Part model, mm, in its own coordinate system. A direction names the side the tool comes from. Round coordinates to 2 decimals unless told otherwise and drop trailing zeros. Write each loop counter-clockwise with the first axis right and the second up, starting at its lowest first coordinate (ties: lowest second). Pieces come first, ordered by that corner, then holes. Notation, with made-up numbers: M 32,81 L 41,81 A11 ccw 41,90 Z; hole C 26,-16.5 d10. An arc over 180 degrees is marked long. One line per question, with ' | ' between items. Start each with the question number.
1) Tool access for faces 4 (the face through (6.46, 2.75, 0.99)), 5 (the face through (0, 2, 1)), 6 (the face through (7.5, 5, 1)): list every direction of +Z, -Z, +X, -X, +Y, -Y with a clear straight run to the whole face (end or side of a thin tool).
2) Saw through at B-B (y = 4). List the corners of the cut face in (x, z).
3) Drop flat-ended pins along their axis: pin 1 Ø0.5 at (y, z) = (5.5, 0.5) entering from +X; pin 2 Ø0.6 at (x, z) = (-0.5, 1) entering from -Y; pin 3 Ø1.1 at (y, z) = (5.5, 1.5) entering from -X; pin 4 Ø1.5 at (x, y) = (-6.5, 4) entering from +Z. Give the stop position or say it passes through.
4) Wall check: probe 1 along X at (y, z) = (4, 1.45); probe 2 along X at (y, z) = (3.2, 1.5); probe 3 along Y at (x, z) = (-2.75, 1.85). Give the ranges that are in metal, low to high. Write a range as [from, to].
5) Saw through at D-D (x = 3.5). List the corners of the cut face in (y, z).
6) Mould opens along X. For faces 1 (the face through (-3.75, 1, 1)), 2 (the face through (0, 3, 2)), 3 (the face through (9.699, 5.465, 1.014)) say: pulls with the +X half, pulls with the -X half, needs draft (parallel to the pull), parting line crosses it, or undercut.
7) Saw through at A-A (y = 1.35). List the corners of the cut face in (x, z).
8) Saw through at C-C (z = 1.15). List the corners of the cut face in (x, y).
```python
from build123d import *

# Parameters (mm, degrees)
TUBE_PLATE_BODY_DEPTH   = 2
TUBE_PLATE_CONTOURING_R = 1


with BuildPart() as part:
    # Sketch1 → Tube Plate Body (new body)
    with BuildSketch(Plane.XY):
        with BuildLine():
            Line((-10, 0), (-10, 5.75))
            Line((-10, 5.75), (-7.5, 5.75))
            Line((-7.5, 5.75), (-7.5, 4.75))
            ThreePointArc((-7.5, 4.75), (-6.5, 2.75), (-5.5, 4.75))
            Line((-5.5, 4.75), (-5.5, 5.75))
            Line((-5.5, 5.75), (5.5, 5.75))
            Line((5.5, 5.75), (5.5, 4.75))
            ThreePointArc((5.5, 4.75), (6.5, 2.75), (7.5, 4.75))
            Line((7.5, 4.75), (7.5, 5.75))
            Line((7.5, 5.75), (10, 5.75))
            Line((10, 5.75), (10, 0))
            Line((10, 0), (3.75, 0))
            Line((3.75, 0), (3.75, 2))
            Line((3.75, 2), (-3.75, 2))
            Line((-3.75, 2), (-3.75, 0))
            Line((-3.75, 0), (-10, 0))
        make_face()
    extrude(amount=TUBE_PLATE_BODY_DEPTH)

    # Tube Plate Contouring
    tube_plate_contouring_edges = [part.edges().sort_by_distance(p)[0] for p in [
        (-10, 5.75, 1),
        (10, 5.75, 1),
    ]]
    fillet(tube_plate_contouring_edges, radius=TUBE_PLATE_CONTOURING_R)


solid = part.part
```
Answer key:
1) face 4: +Z, -Z | face 5: +Z, -Z, -Y | face 6: +Z, -Z, +Y
2) outline: M -10,0 L -7.75,0 L -7.75,2 L -10,2 Z; M -5.25,0 L 5.25,0 L 5.25,2 L -5.25,2 Z; M 7.75,0 L 10,0 L 10,2 L 7.75,2 Z
3) pin 1: stops at x = 9.87 | pin 2: stops at y = 2 | pin 3: stops at x = -9.98 | pin 4: passes through
4) probe 1: x = [-10, -7.75], [-5.25, 5.25], [7.75, 10] | probe 2: x = [-10, -7.46], [-5.54, 5.54], [7.46, 10] | probe 3: y = [2, 5.75]
5) outline: M 2,0 L 5.75,0 L 5.75,2 L 2,2 Z
6) face 1: undercut | face 2: needs draft | face 3: pulls with the +X half
7) outline: M -10,0 L -3.75,0 L -3.75,2 L -10,2 Z; M 3.75,0 L 10,0 L 10,2 L 3.75,2 Z
8) outline: M -10,0 L -3.75,0 L -3.75,2 L 3.75,2 L 3.75,0 L 10,0 L 10,4.75 A1 ccw 9,5.75 L 7.5,5.75 L 7.5,4.75 A1.25 cw long 5.5,4.75 L 5.5,5.75 L -5.5,5.75 L -5.5,4.75 A1.25 cw long -7.5,4.75 L -7.5,5.75 L -9,5.75 A1 ccw -10,4.75 Z
